The listing builds one solid part. Answer for the finished solid, in the listing's coordinates (mm). Face numbers are marked on the shaded views. Give positions to 0.01 mm unless a question says otherwise; leave off trailing zeros. Write each loop counter-clockwise with the first axis right and the second up, starting at its lowest first coordinate (ties: lowest second). Pieces come first, ordered by that corner, then holes. Notation, with made-up numbers: M 35.25,46.5 L 51.25,46.5 A20 cw 51.25,64.5 Z; hole C -26,6 d9. An arc over 180 degrees is marked long. Answer as a JSON object with one key per item and string values.
```python
from build123d import *

# Parameters (mm, degrees)
F3_DEPTH  = 2.032
F4_DEPTH  = 1.016
F5_DEPTH  = 2.032
F6_SCALE  = 0.5
F7_DEPTH  = 12.7
F10_DEPTH = 25.4


with BuildPart() as f3:
    # F0 (on Front) → F3 (new body)
    with BuildSketch(Plane.XZ):
        Polygon((1.7399819335, 32.9988971353), (-12.4273560941, 32.9988971353), (-18.1648561832, 21.6064513681), (1.4037427613, 21.6064513681), (0.6089702947, 20.0053038526), (-18.9712312321, 20.0053038526), (-20.7453668118, 16.4825599641), (6.9015445188, 16.4825599641), (11.0007077456, 24.8590362167), (-8.4278472578, 24.8590362167), (-6.8397070281, 28.0124656121), (-0.7713007088, 28.0124656121), align=None)
    extrude(amount=F3_DEPTH)


with BuildPart() as f3b:
    # F0 (on Front) → F3, piece 2 (new body)
    with BuildSketch(Plane.XZ):
        Polygon((15.0998709723, 32.9988971353), (6.9015445188, 32.9988971353), (4.449058262, 28.0581217034), (12.6473847156, 28.0581217034), align=None)
    extrude(amount=F3_DEPTH)


with BuildPart() as f4:
    # F1 (on Front) → F4 (new body)
    with BuildSketch(Plane.XZ):
        Polygon((-14.3832698171, 36.1738971353), (-25.8992879083, 13.3075599641), (8.8825950149, 13.3075599641), (20.0726044695, 36.1738971353), align=None)
    extrude(amount=F4_DEPTH)

    # F2 (on Front) → F5 (join)
    with BuildSketch(Plane.XZ):
        Polygon((-15.9480007955, 38.7138971353), (-30.0224247855, 10.7675599641), (10.4674354118, 10.7675599641), (24.1434244793, 38.7138971353), align=None)
        Polygon((20.0726044695, 36.1738971353), (8.8825950149, 13.3075599641), (-25.8992879083, 13.3075599641), (-14.3832698171, 36.1738971353), align=None, mode=Mode.SUBTRACT)
    extrude(amount=F5_DEPTH)


with BuildPart() as f4_1:
    # F6: moved
    add(f4.part.scale(F6_SCALE).moved(Location((-3.4198535141, 0, 14.0062328061))))


with BuildPart() as f3_1:
    # F6: moved
    add(f3.part.scale(F6_SCALE).moved(Location((-3.4198535141, 0, 14.0062328061))))

    # F7 (add): a face of the model
    f7_faces = [f4_1.part.faces().sort_by_distance(p)[0] for p in [
        (-4.8455163994, 0, 26.3650820037),
    ]]


with BuildPart() as f3b_1:
    # F6: moved
    add(f3b.part.scale(F6_SCALE).moved(Location((-3.4198535141, 0, 14.0062328061))))


with BuildPart() as f3_2:
    add(f3_1.part)

    add(f3b_1.part)  # F7 merges F3b

    add(f4_1.part)  # F7 merges F4
    extrude(f7_faces, amount=F7_DEPTH)

    # F9 (on face) → F10 (cut)
    with BuildSketch(Plane.XY.offset(33.3631813737)):
        with BuildLine():
            ThreePointArc((-4.8896035063, 0), (22.0511648024, 11.1592316666), (33.2103964094, 38.1))
            ThreePointArc((33.2103964094, 38.1), (-31.8303719836, 65.0407683334), (-4.8896035063, 0))
        make_face()
    extrude(amount=-F10_DEPTH, mode=Mode.SUBTRACT)


solid = f3_2.part
```
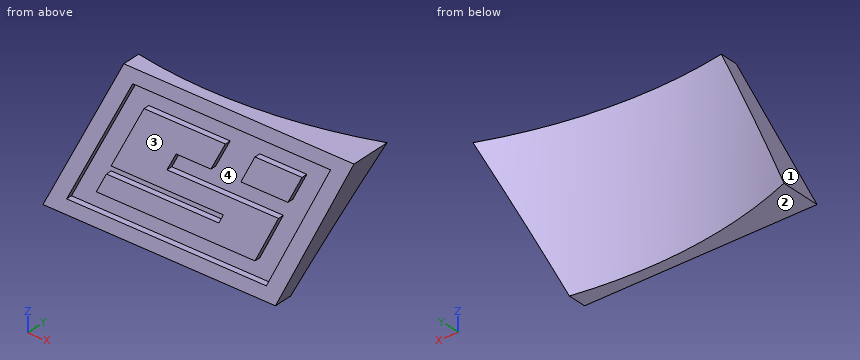
1. A cutting plane is placed at B-B, the plane z = 26. Give the vertices of the cut face in (x, y).
Verdict:
{"outline": "M -15.1,-1.02 L -13.68,-1.02 L -13.68,-0.51 L -11.9,-0.51 L -11.9,-1.02 L 1.87,-1.02 L 1.87,-0.51 L 3.63,-0.51 L 3.63,-1.02 L 5.05,-1.02 L 5.05,1.32 A38.1 cw -15.1,1.39 Z"}
2. Flat-ended cylindrical pins translate along their axes: pin 1 (1 mm diameter, centred on y = 0.5, z = 21, fed in from -X); pin 2 (6 mm diameter, centred on x = -13.5, z = 29, fed in from +Y); pin 3 (5 mm diameter, centred on x = -13.5, z = 25, fed in from +Y). Find the tip coordinate at first contact, or state that the pin passes through.
Verdict:
{"pin 1": "stops at x = -17.87", "pin 2": "stops at y = 1.34", "pin 3": "stops at y = 1.63"}
3. A cutting plane is placed at A-A, the plane y = 1.7. Give the vertices of the cut face in (x, z), plus the area to 3 significant figures.
Verdict:
{"outline": "M -18.43,19.39 L -16.14,19.39 L -16.14,23.93 Z; M 6.36,28.69 L 8.65,33.36 L 6.36,33.36 Z", "area": "10.5 mm2"}
4. A cutting plane is placed at C-C, the plane x = 5.5. Give the vertices of the cut face in (y, z).
Verdict:
{"outline": "M -1.02,26.92 L 1.44,26.92 L 1.44,33.36 L -1.02,33.36 L -1.02,32.09 L -0.51,32.09 L -0.51,29.81 L -1.02,29.81 Z"}
5. The mould has two halves that part along Z. Classify the marked faces 1, 2, 3 and 4: released by +Z, released by -Z, zero draft, split by the parting line, or undercut.
Verdict:
{"face 1": "released by +Z", "face 2": "released by -Z", "face 3": "zero draft", "face 4": "undercut"}
6. Consider line 1 along Y through (x, z) = (-5, 32.5); line 2 along Z through (x, y) = (-15.25, -0.6); line 3 along Y through (x, z) = (-4.25, 24.25). Determine where each line is inside the solid, lowest interval first.
Verdict:
{"line 1": "y = -1.02 to 0", "line 2": "z = 19.39 to 20.66, 22.88 to 25.71", "line 3": "y = -0.51 to 0.01"}
7. A cutting plane is placed at D-D, the plane x = -14.5. Give the vertices of the cut face in (y, z), plus the area to 3 significant figures.
Verdict:
{"outline": "M -1.02,19.39 L 1.23,19.39 L 1.23,27.2 L -1.02,27.2 L -1.02,24.37 L -0.51,24.37 L -0.51,20.66 L -1.02,20.66 Z", "area": "15.7 mm2"}
